```python
from build123d import *

# Parameters (mm, degrees)
F0_R     = 19.05
F1_DEPTH = 25.4
F2_T     = -1.27
F3_R     = 2.54
F3_R_2   = 19.05
F4_DEPTH = 2.54
F5_R     = 1.27
F6_DEPTH = 7.62


with BuildPart() as f1:
    # F0 (on Top) → F1 (new body)
    with BuildSketch(Plane.XY):
        Circle(F0_R)
    extrude(amount=F1_DEPTH)

    # F2
    f2_openings = [f1.faces().sort_by_distance(p)[0] for p in [
        (0, 0, 25.4),
    ]]
    offset(amount=F2_T, openings=f2_openings)

    # F3 (on face) → F4 (join)
    with BuildSketch(Plane(origin=(0, 0, 0), x_dir=(1, 0, 0), z_dir=(0, 0, -1))):
        with BuildLine():
            ThreePointArc((-20.6561764706, 6.2809612016), (-27.94, 0), (-20.6561764706, -6.2809612016))
            ThreePointArc((-20.6561764706, -6.2809612016), (21.59, 0), (-20.6561764706, 6.2809612016))
        make_face()
        with Locations((-23.495, 0)):
            Circle(F3_R, mode=Mode.SUBTRACT)
        Circle(F3_R_2, mode=Mode.SUBTRACT)
    extrude(amount=-F4_DEPTH)

    # F5 (on face) → F6 (join)
    with BuildSketch(Plane.XY.offset(1.27)):
        Circle(F5_R)
    extrude(amount=F6_DEPTH)


solid = f1.part
```
Part model, mm, in its own coordinate system. A direction names the side the tool comes from. Coordinates: 2 decimals unless noted, no trailing zeros. Order: outer loops, then holes, each group sorted by start corner. A loop starts at its lowest first (then second) coordinate and runs counter-clockwise, first axis right, second up. Notation, with made-up numbers: (69, 31) - (124, 31) arc R4 cw to (124, 36) - close; hole circle Ø3 at (77.25, 1). An arc over 180 degrees is marked (long way). Return JSON: item names as keys, results as strings. Group by question number.
Item 1: Pin check, flat tips, straight feed: pin 1 (5 mm diameter, centred on y = 4, z = 16.5, fed in from -X); pin 2 (2 mm diameter, centred on x = 0, y = 0.5, fed in from +Z); pin 3 (2 mm diameter, centred on y = -5.5, z = 16, fed in from -X). Stop position of each tip, or through.
Item 2: Cut at A-A (y = 0). List the corners of the cut face in (x, z) (3 decimals), plus the area to 3 significant figures.
Item 3: Cut at B-B (z = 4.75). List the corners of the cut face in (x, y), plus the area to 3 significant figures.
Item 4: Cut at C-C (x = -21.59). List the corners of the cut face in (y, z).
Item 5: Drill centre lines: probe 1 along Y at (x, z) = (0.5, 19.25); probe 2 along Z at (x, y) = (3, 0.5); probe 3 along Z at (x, y) = (8.5, 18). Where is each one in solid material? Low to high. Write a range as from..to.
Item 6: Which spindle directions (+Z, -Z, +X, -X, +Y, -Y) get a long thin tool onto all of the face, cutting with end or side? Do faces 1 (the face through (-26.033, -0.112, 1.252)), 2 (the face through (-20, 0, 2.54)). Say none if no direction does.
Item 7: Cut at D-D (x = 0). List the corners of the cut face in (y, z), plus the area to 3 significant figures.
Item 8: Pull direction Y, two halves, no side cores. Call faces 3 (the face through (-3.85, -17.36, 13.17)), 4 (the face through (-16, 9, 25.4)), 5 (the face through (21.573, 0.86, 1.252)): pulls with the +Y half, pulls with the -Y half, needs draft (parallel to the pull), parting line crosses it, or undercut.
Check values:
{
 "1": {"pin 1": "stops at x = -18.99", "pin 2": "stops at z = 8.89", "pin 3": "stops at x = -18.51"},
 "2": {"outline": "(-27.94, 0) - (-26.035, 0) - (-26.035, 2.54) - (-27.94, 2.54) - close; (-20.955, 0) - (21.59, 0) - (21.59, 2.54) - (19.05, 2.54) - (19.05, 25.4) - (17.78, 25.4) - (17.78, 1.27) - (1.27, 1.27) - (1.27, 8.89) - (-1.27, 8.89) - (-1.27, 1.27) - (-17.78, 1.27) - (-17.78, 25.4) - (-19.05, 25.4) - (-19.05, 2.54) - (-20.955, 2.54) - close", "area": "145 mm2"},
 "3": {"outline": "circle Ø38.1 at (0, 0); circle Ø2.54 at (0, 0); hole circle Ø35.56 at (0, 0)", "area": "152 mm2"},
 "4": {"outline": "(-6.35, 0) - (-1.68, 0) - (-1.68, 2.54) - (-6.35, 2.54) - close; (1.68, 0) - (6.35, 0) - (6.35, 2.54) - (1.68, 2.54) - close"},
 "5": {"probe 1": "y = -19.04..-17.77, 17.77..19.04", "probe 2": "z = 0..1.27", "probe 3": "z = 0..2.54"},
 "6": {"face 1": "+Z, -Z", "face 2": "+Z"},
 "7": {"outline": "(-21.59, 0) - (21.59, 0) - (21.59, 2.54) - (19.05, 2.54) - (19.05, 25.4) - (17.78, 25.4) - (17.78, 1.27) - (1.27, 1.27) - (1.27, 8.89) - (-1.27, 8.89) - (-1.27, 1.27) - (-17.78, 1.27) - (-17.78, 25.4) - (-19.05, 25.4) - (-19.05, 2.54) - (-21.59, 2.54) - close", "area": "142 mm2"},
 "8": {"face 3": "undercut", "face 4": "needs draft", "face 5": "parting line crosses it"}
}
